Job drawing, mm, ordinate dimensions from the low corner. One solid piece. A direction names the side the tool comes from. Give positions to 0.01 mm unless a question says otherwise; leave off trailing zeros. Loops run counter-clockwise (first coordinate to the right, second up) from the corner with the lowest first, then second, coordinate; pieces in that order, holes last. Notation, with made-up numbers: M 27,23 L 83,23 A16 ccw 83,31 Z; hole C 37.25,17 d5. An arc over 180 degrees is marked long. One line per question, with ' | ' between items.
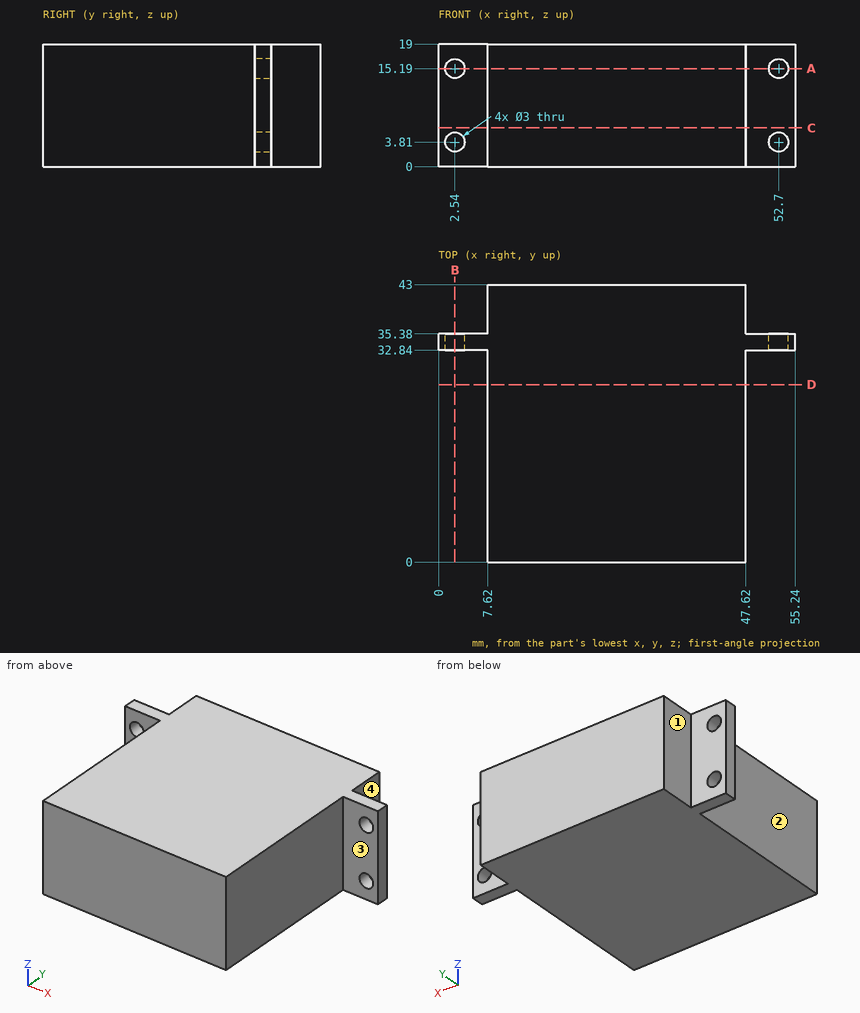
Item 1: Saw through at C-C on z = 6. Give the cut face in (x, y).
Conclusion:
outline: M 0,32.84 L 7.62,32.84 L 7.62,0 L 47.62,0 L 47.62,32.84 L 55.24,32.84 L 55.24,35.38 L 47.62,35.38 L 47.62,43 L 7.62,43 L 7.62,35.38 L 0,35.38 Z
Item 2: Saw through at A-A on z = 15.19. Give the cut face in (x, y).
Conclusion:
outline: M 0,32.84 L 1.04,32.84 L 1.04,35.38 L 0,35.38 Z; M 4.04,32.84 L 7.62,32.84 L 7.62,0 L 47.62,0 L 47.62,32.84 L 51.2,32.84 L 51.2,35.38 L 47.62,35.38 L 47.62,43 L 7.62,43 L 7.62,35.38 L 4.04,35.38 Z; M 54.2,32.84 L 55.24,32.84 L 55.24,35.38 L 54.2,35.38 Z
Item 3: 3-axis set-ups, long thin cutter, end or side, ignore diameter. For the marked faces 1, 2, 3 and 4: which of +Z, -Z, +X, -X, +Y, -Y reach the whole face in a straight line?
Conclusion:
face 1: +Z, -Z, -X, +Y | face 2: +Z, -Z, -X, -Y | face 3: +Z, -Z, +X, -Y | face 4: +Z, -Z, +X, +Y
Item 4: Saw through at D-D on y = 27.5. Give the cut face in (x, z).
Conclusion:
outline: M 7.62,0 L 47.62,0 L 47.62,19 L 7.62,19 Z
Item 5: Drill centre lines: line 1 along X through (y, z) = (34.75, 15.19); line 2 along Z through (x, y) = (52.7, 34.6); line 3 along X through (y, z) = (34, 15.75). Where is each one in solid material? Low to high. Write a range as [from, to].
Conclusion:
line 1: [0, 1.04], [4.04, 51.2], [54.2, 55.24] | line 2: [0, 2.31], [5.31, 13.69], [16.69, 19] | line 3: [0, 1.15], [3.93, 51.31], [54.09, 55.24]
Item 6: Drop flat-ended pins along their axis: P1, Ø4, axis at y = 19.5, z = 7, coming from the +X side; P2, Ø6, axis at x = 52, z = 13, coming from the -Y side; P3, Ø2.5, axis at x = 3.5, z = 10, coming from the +Y side; P4, Ø1.5, axis at x = 27.5, z = 5, coming from the -Y side. Give the stop position or say it passes through.
Conclusion:
P1: x = 47.62 | P2: y = 32.84 | P3: y = 35.38 | P4: y = 0
Item 7: Saw through at B-B on x = 2.54. Give the cut face in (y, z), and give its area (3 significant figures).
Conclusion:
outline: M 32.84,0 L 35.38,0 L 35.38,2.31 L 32.84,2.31 Z; M 32.84,5.31 L 35.38,5.31 L 35.38,13.69 L 32.84,13.69 Z; M 32.84,16.69 L 35.38,16.69 L 35.38,19 L 32.84,19 Z | area: 33.0 mm²
